Source: CAD feature listing. Evaluate the final solid. Frame: model axes, mm. A direction names the side the tool comes from. Give positions to 0.01 mm unless a question says otherwise; leave off trailing zeros. Order: outer loops, then holes, each group sorted by start corner. A loop starts at its lowest first (then second) coordinate and runs counter-clockwise, first axis right, second up. Notation, with made-up numbers: M 31.5,-35.75 L 50.5,-35.75 A9 cw 50.5,-18.75 Z; hole C 52.25,16 d4. An arc over 180 degrees is marked long. Return JSON: item names as keys, results as strings.
from build123d import *

# Parameters (mm, degrees)
F0_R     = 41.275
F1_DEPTH = 9.525
F0_R_2   = 25.4
F2_DEPTH = 38.1
F0_R_3   = 15.875
F3_DEPTH = 19.05
F4_R     = 25.4


with BuildPart() as f1:
    # F0 (on Top) → F1 (new body, symmetric)
    with BuildSketch(Plane.XY):
        with BuildLine():
            Line((-215.7407249902, -87.2876721291), (8.4498648325, -46.8693973645))
            ThreePointArc((8.4498648325, -46.8693973645), (-32.7711116329, -34.5571246973), (-47.251464821, 5.953125))
            Line((-47.251464821, 5.953125), (-43.6005938779, 34.9310147533))
            Line((-43.6005938779, 34.9310147533), (-230.4807845369, -32.277020994))
            ThreePointArc((-230.4807845369, -32.277020994), (-204.3758278578, -35.7902460874), (-192.2356438897, -59.1660337104))
            ThreePointArc((-192.2356438897, -59.1660337104), (-198.885731603, -77.4916672936), (-215.7407249902, -87.2876721291))
        make_face()
        with BuildLine():
            ThreePointArc((-47.251464821, 5.953125), (-37.1678516079, 29.7773644208), (-16.1169010787, 44.815021194))
            Line((-16.1169010787, 44.815021194), (-43.6005938779, 34.9310147533))
            Line((-43.6005938779, 34.9310147533), (-47.251464821, 5.953125))
        make_face()
        with BuildLine():
            ThreePointArc((8.4498648325, -46.8693973645), (36.5415204777, -30.5427226385), (47.625, 0))
            ThreePointArc((47.625, 0), (47.5315244711, 2.9824162099), (47.251464821, 5.953125))
            ThreePointArc((47.251464821, 5.953125), (24.8978314077, 40.598505098), (-16.1169010787, 44.815021194))
            ThreePointArc((-16.1169010787, 44.815021194), (-37.1678516079, 29.7773644208), (-47.251464821, 5.953125))
            ThreePointArc((-47.251464821, 5.953125), (-32.7711116329, -34.5571246973), (8.4498648325, -46.8693973645))
        make_face()
        Circle(F0_R, mode=Mode.SUBTRACT)
        with BuildLine():
            ThreePointArc((-16.1169010787, 44.815021194), (24.8978314077, 40.598505098), (47.251464821, 5.953125))
            Line((47.251464821, 5.953125), (28.3508788926, 155.971875))
            ThreePointArc((28.3508788926, 155.971875), (28.5189146827, 154.1894497259), (28.575, 152.4))
            ThreePointArc((28.575, 152.4), (-1.7894497259, 123.8810853173), (-28.3508788926, 155.971875))
            Line((-28.3508788926, 155.971875), (-43.6005938779, 34.9310147533))
            Line((-43.6005938779, 34.9310147533), (-16.1169010787, 44.815021194))
        make_face()
    extrude(amount=F1_DEPTH, both=True)

    # F0 (on Top) → F2 (join, symmetric)
    with BuildSketch(Plane.XY):
        Circle(F0_R)
        Circle(F0_R_2, mode=Mode.SUBTRACT)
    extrude(amount=F2_DEPTH, both=True)

    # F0 (on Top) → F3 (join, symmetric)
    with BuildSketch(Plane.XY):
        with BuildLine():
            ThreePointArc((-230.4807845369, -32.277020994), (-248.4119743759, -66.5617879242), (-215.7407249902, -87.2876721291))
            ThreePointArc((-215.7407249902, -87.2876721291), (-198.885731603, -77.4916672936), (-192.2356438897, -59.1660337104))
            ThreePointArc((-192.2356438897, -59.1660337104), (-204.3758278578, -35.7902460874), (-230.4807845369, -32.277020994))
        make_face()
        with Locations((-220.8106438897, -59.1660337104)):
            Circle(F0_R_3, mode=Mode.SUBTRACT)
        with BuildLine():
            ThreePointArc((28.575, 152.4), (28.5189146827, 154.1894497259), (28.3508788926, 155.971875))
            ThreePointArc((28.3508788926, 155.971875), (0, 180.975), (-28.3508788926, 155.971875))
            ThreePointArc((-28.3508788926, 155.971875), (-1.7894497259, 123.8810853173), (28.575, 152.4))
        make_face()
        with Locations((0, 152.4)):
            Circle(F0_R_3, mode=Mode.SUBTRACT)
    extrude(amount=F3_DEPTH, both=True)

    # F4
    f4_edges = [f1.edges().sort_by_distance(p)[0] for p in [
        (-43.600594, 34.931015, 0),
    ]]
    fillet(f4_edges, radius=F4_R)


solid = f1.part
1. Section query B-B (x = 0). Return loops of the section in (y, z) (3 decimals), then the cut area to 3 significant figures.
Evaluation:
{"outline": "M -48.393,-9.525 L -41.275,-9.525 L -41.275,-38.1 L -25.4,-38.1 L -25.4,38.1 L -41.275,38.1 L -41.275,9.525 L -48.393,9.525 Z; M 25.4,-38.1 L 41.275,-38.1 L 41.275,-9.525 L 123.825,-9.525 L 123.825,-19.05 L 136.525,-19.05 L 136.525,19.05 L 123.825,19.05 L 123.825,9.525 L 41.275,9.525 L 41.275,38.1 L 25.4,38.1 Z; M 168.275,-19.05 L 180.975,-19.05 L 180.975,19.05 L 168.275,19.05 Z", "area": "5,100 mm^2"}
2. Section query A-A (y = 0). Return loops of the section in (x, z) (3 decimals).
Evaluation:
{"outline": "M -140.731,-9.525 L -41.275,-9.525 L -41.275,-38.1 L -25.4,-38.1 L -25.4,38.1 L -41.275,38.1 L -41.275,9.525 L -140.731,9.525 Z; M 25.4,-38.1 L 41.275,-38.1 L 41.275,-9.525 L 47.625,-9.525 L 47.625,9.525 L 41.275,9.525 L 41.275,38.1 L 25.4,38.1 Z"}
3. Section query C-C (z = -32.5). Return loops of the section in (x, y) (3 decimals), then the cut area to 3 significant figures.
Evaluation:
{"outline": "C 0,0 d82.55; hole C 0,0 d50.8", "area": "3,330 mm^2"}
4. Ray query, probe 1 along Y at (x, z) = (0, 5) (3 decimals); probe 2 along Z at (x, y) = (-34.5, 42.5) (3 decimals); probe 3 along Y at (x, z) = (-142, -6.5). Return the intervals inside material, ascending.
Evaluation:
{"probe 1": "y = -48.393 to -25.4, 25.4 to 136.525, 168.275 to 180.975", "probe 2": "z = -9.525 to 9.525", "probe 3": "y = -73.99 to -0.46"}
5. Set-up query: faces 1 (the face through (-61, 8, 9.525)), 2 (the face through (12, 140, -19.05)), 3 (the face through (-209, -71, -19.05)), 4 (the face through (12, 140, 19.05)). Return all of +Z, -Z, +X, -X, +Y, -Y with unobstructed straight access to the full face (end or side cutting, diameter ignored); none if empty.
Evaluation:
{"face 1": "+Z", "face 2": "-Z, +X, -X, +Y", "face 3": "-Z, -X, +Y, -Y", "face 4": "+Z, +X, -X, +Y"}
6. Section query D-D (y = 152.4). Return loops of the section in (x, z) (3 decimals), then the cut area to 3 significant figures.
Evaluation:
{"outline": "M -28.801,-9.525 L -28.575,-9.525 L -28.575,-19.05 L -15.875,-19.05 L -15.875,19.05 L -28.575,19.05 L -28.575,9.525 L -28.801,9.525 Z; M 15.875,-19.05 L 28.575,-19.05 L 28.575,-9.525 L 28.801,-9.525 L 28.801,9.525 L 28.575,9.525 L 28.575,19.05 L 15.875,19.05 Z", "area": "976 mm^2"}
7. Draft query along Y for faces 5 (the face through (-61, 8, -9.525)), 6 (the face through (-34.91, 103.92, 0.13)), 7 (the face through (-19, -18, 38.1)). Return one class per face: pulls with the +Y half, pulls with the -Y half, needs draft (parallel to the pull), parting line crosses it, or undercut.
Evaluation:
{"face 5": "undercut", "face 6": "pulls with the +Y half", "face 7": "needs draft"}
8. First-contact query: pin 1 (8 mm diameter, centred on y = 118.5, z = 21.5, fed in from +X); pin 2 (17 mm diameter, centred on x = -7.5, y = 145.5, fed in from +Z); pin 3 (2 mm diameter, centred on x = -97.5, z = 2.5, fed in from +Y); pin 4 (2 mm diameter, centred on x = -28.5, z = 2, fed in from -Y). Flat tips, straight axial feed; report the tip coordinate or a pass-through.
Evaluation:
{"pin 1": "passes through", "pin 2": "stops at z = 19.05", "pin 3": "stops at y = 15.91", "pin 4": "stops at y = -53.71"}
